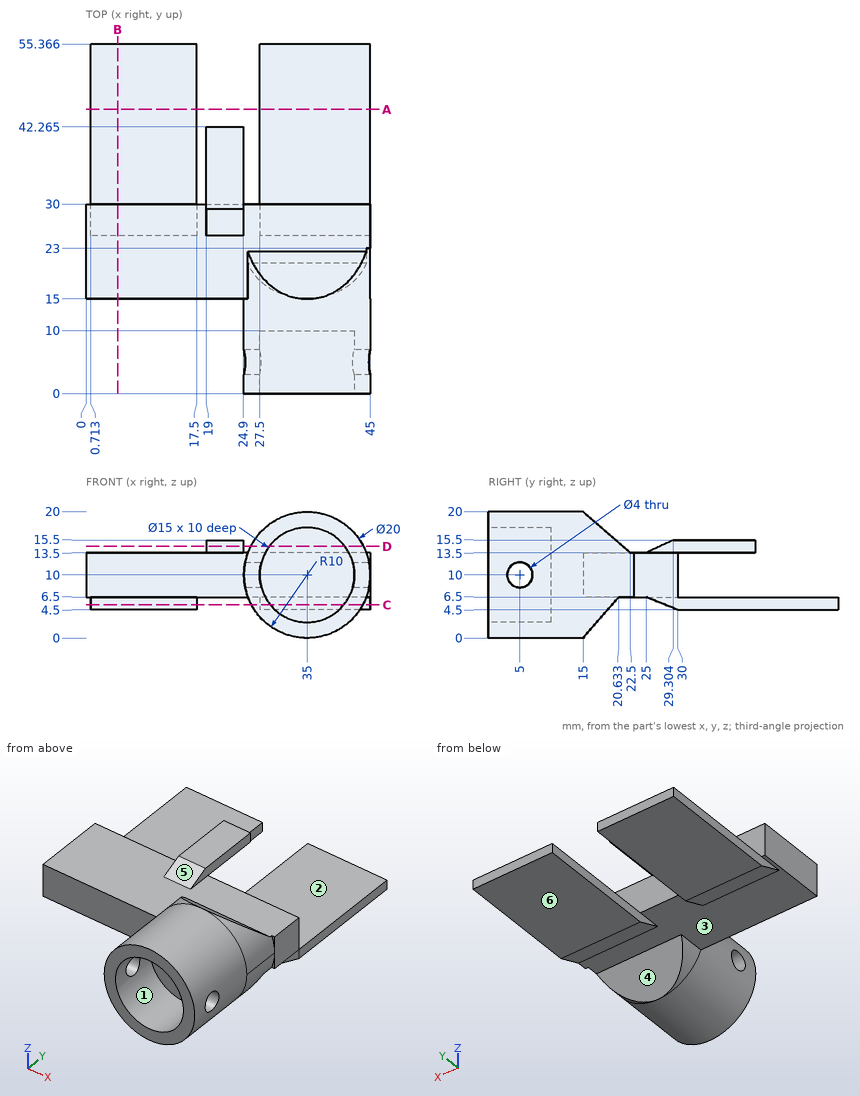
Here's the drawing with two shaded views (mm, measured from the low corner). I have some questions. A direction names the side the tool comes from. Coordinates: 2 decimals unless noted, no trailing zeros. Write each loop counter-clockwise with the first axis right and the second up, starting at its lowest first coordinate (ties: lowest second). Pieces come first, ordered by that corner, then holes. Notation, with made-up numbers: (-30, 53) -> (-20, 53) arc R16 ccw to (-20, 78) -> close; hole circle Ø7 at (-22.75, -39.5). An arc over 180 degrees is marked (long way). Use a Markdown table: item, result. Add a question column.
(1) If we section it at A-A, the plane y = 45: Write out the boundary of the cut face in (x, z).
(2) If we section it at D-D, the plane z = 14.5: Write out the boundary of the cut face in (x, y) (1 decimal).
(3) I'm going to push flat-ended pins straight in: P1, Ø8, axis at y = 47.5, z = 3, coming from the -X side; P2, Ø1.5, axis at x = 5.5, y = 43, coming from the -Z side; P3, Ø2, axis at y = 31.5, z = 14.5, coming from the +X side. Where does each tip first touch, or does it pass through?
(4) We'd pull the mould along Y, two halves only. Please class the marked faces 4, 5 and 6: +Y half, -Y half, draft (parallel to the pull), parting line (faces both ways), or undercut.
(5) For the marked faces 1, 2 and 3, which set-ups out of +Z, -Z, +X, -X, +Y, -Y let a thin tool reach every point of the face, with its end or its side?
(6) If we section it at B-B, the plane x = 5: Write out the boundary of the cut face in (y, z).
(7) If we section it at C-C, the plane z = 5.25: State how many separate pieces and enclosed holes the cut face has, and give its area (3 significant figures).
(8) Please list where these lines run through material, in increasing order: line 1 (X direction, y = 48, z = 5); line 2 (Z direction, x = 8, y = 47); line 3 (Z direction, x = 21, y = 41).
Outcome:
| question | item | result |
|---|---|---|
| 1 | outline | (0.71, 4.5) -> (17.5, 4.5) -> (17.5, 6.5) -> (0.71, 6.5) -> close; (27.5, 4.5) -> (45, 4.5) -> (45, 6.5) -> (27.5, 6.5) -> close |
| 2 | outline | (19, 27.2) -> (24.9, 27.2) -> (24.9, 42.3) -> (19, 42.3) -> close; (26.1, 0) -> (29, 0) -> (29, 10) -> (41, 10) -> (41, 0) -> (43.9, 0) -> (43.9, 21.3) -> (26.1, 21.3) -> close |
| 3 | P1 | stops at x = 0.71 |
| 3 | P2 | stops at z = 4.5 |
| 3 | P3 | stops at x = 24.9 |
| 4 | face 4 | undercut |
| 4 | face 5 | -Y half |
| 4 | face 6 | draft |
| 5 | face 1 | -Y |
| 5 | face 2 | +Z, +X, -X, +Y |
| 5 | face 3 | -Z |
| 6 | outline | (15, 6.5) -> (25, 6.5) -> (30, 4.5) -> (55.37, 4.5) -> (55.37, 6.5) -> (30, 6.5) -> (30, 13.5) -> (15, 13.5) -> close |
| 7 | separate pieces | 3 |
| 7 | enclosed holes | 0 |
| 7 | area | 1,160 mm^2 |
| 8 | line 1 | x = 0.71 to 17.5, 27.5 to 45 |
| 8 | line 2 | z = 4.5 to 6.5 |
| 8 | line 3 | z = 13.5 to 15.5 |
